Autodesk Fusion 360 part; units mm, degrees
sketch "Sketch1" plane through (0, 0, 0) normal (0, 0, 1) x (1, 0, 0)
  line L0 (-41.2185, 94.5561) -> (-4.3961, 94.5561)
  line L1 (-4.3961, 94.5561) -> (-4.3961, -73.6817)
  line L2 (-4.3961, -73.6817) -> (-41.2185, -73.6817)
  line L3 (-41.2185, -73.6817) -> (-41.2185, 94.5561)
  line L4 (84.0952, 92.7118) -> (116.424, 75.0841)
  line L5 (116.424, 75.0841) -> (35.8844, -72.6229)
  line L6 (35.8844, -72.6229) -> (3.5557, -54.9951)
  line L7 (3.5557, -54.9951) -> (84.0952, 92.7118)
  line L8 (81.0854, 27.7563) -> (81.0854, -6.6095)
  line L9 (81.0854, -6.6095) -> (-34.3246, -6.6095)
  line L10 (-34.3246, -6.6095) -> (-34.3246, 27.7563)
  line L11 (-34.3246, 27.7563) -> (81.0854, 27.7563)
extrude "Extrude2" add sketch "Sketch1" along normal blind 48 contours L1 L7 L9 L11 | L1 L9 L10 L11 | L5 L7 L8 L9 L11 | L5 L8 L9 makes body 1
extrude "Extrude1" add sketch "Sketch1" along normal blind 38 separate body contours L0 L1 L2 L3 L9 L10 L11 makes body 2
extrude "Extrude3" add sketch "Sketch1" along normal blind 38 separate body contours L5 L6 L7 L9 makes body 3
extrude "Extrude4" add sketch "Sketch1" along normal blind 38 separate body contours L4 L5 L7 L8 L11 makes body 4
combine "Combine1" operation add target body 4 tool bodies 3 2 1
Input: part model. Units: mm. Frame: model coordinates. A direction names the side the tool comes from. Coordinates: 2 decimals unless noted, no trailing zeros. Write each loop counter-clockwise with the first axis right and the second up, starting at its lowest first coordinate (ties: lowest second). Pieces come first, ordered by that corner, then holes. Notation, with made-up numbers: M 40.5,81 L 88.5,81 A17 ccw 88.5,95 Z; hole C -20.5,58 d3. An arc over 180 degrees is marked long. Use one line per item in the form item = value.
Q1. Section D-D (x = -26.5). Return loops of the section in (y, z), plus the area to 3 significant figures.
Answer below:
outline = M -73.68,0 L 94.56,0 L 94.56,38 L 27.76,38 L 27.76,48 L -6.61,48 L -6.61,38 L -73.68,38 Z
area = 6,740 mm²
Q2. Section C-C (z = 10.5). Return loops of the section in (x, y), plus the area to 3 significant figures.
Answer below:
outline = M -41.22,-73.68 L -4.4,-73.68 L -4.4,-6.61 L 29.94,-6.61 L 3.56,-55 L 35.88,-72.62 L 71.88,-6.61 L 81.09,-6.61 L 81.09,10.27 L 116.42,75.08 L 84.1,92.71 L 48.68,27.76 L -4.4,27.76 L -4.4,94.56 L -41.22,94.56 Z
area = 14,000 mm²
Q3. First-contact query: pin 1 (5 mm diameter, centred on x = 47.5, z = 12.5, fed in from -Y); pin 2 (3 mm diameter, centred on y = 2, z = 43.5, fed in from -X); pin 3 (24 mm diameter, centred on x = 40.5, z = 28, fed in from -Y). Flat tips, straight axial feed; report the tip coordinate or a pass-through.
Answer below:
pin_1 = -55.91
pin_2 = -34.32
pin_3 = -72.62
Q4. Set-up query: faces 5 (the face through (19.946, -63.932, 18.734)), 6 (the face through (16.563, -31.141, 18.734)), 7 (the face through (81.085, 3, 29)), 8 (the face through (66.14, 59.78, 18.73)). Return all of +Z, -Z, +X, -X, +Y, -Y with unobstructed straight access to the full face (end or side cutting, diameter ignored); none if empty.
Answer below:
face_5 = +Z, -Z, -Y
face_6 = +Z, -Z
face_7 = +Z, +X, -Y
face_8 = +Z, -Z, +Y
Q5. Section B-B (y = 63). Return loops of the section in (x, z), plus the area to 3 significant figures.
Answer below:
outline = M -41.22,0 L -4.4,0 L -4.4,38 L -41.22,38 Z; M 67.89,0 L 109.83,0 L 109.83,38 L 67.89,38 Z
area = 2,990 mm²
Q6. Draft query along X for faces 1 (the face through (54.134, -39.154, 18.734)), 2 (the face through (-4.396, 62, 19)), 3 (the face through (-34.325, 10, 43)), 4 (the face through (24, -6.61, 29)). Return one class per face: released by +X, released by -X, zero draft, split by the parting line, or undercut.
Answer below:
face_1 = released by +X
face_2 = undercut
face_3 = released by -X
face_4 = undercut
Q7. Material intervals for probe 1 along Z at (x, y) = (33.5, -27.5); probe 2 along Y at (x, z) = (14.5, 22); probe 3 along Y at (x, z) = (73.5, 41.5), sorted ascending. Write a range as from..to.
Answer below:
probe_1 = 0..38
probe_2 = -60.96..-34.92, -6.61..27.76
probe_3 = -6.61..27.76
Q8. Section A-A (x = 14). Return loops of the section in (y, z).
Answer below:
outline = M -60.69,0 L -35.84,0 L -35.84,38 L -60.69,38 Z; M -6.61,0 L 27.76,0 L 27.76,48 L -6.61,48 Z
